CAD build for the part. Positions are in the model's coordinates, mm. A direction names the side the tool comes from. Coordinates: 2 decimals unless noted, no trailing zeros. Order: outer loops, then holes, each group sorted by start corner. A loop starts at its lowest first (then second) coordinate and runs counter-clockwise, first axis right, second up. Notation, with made-up numbers: (34, 0.5) - (88, 0.5) arc R8 cw to (88, 4.5) - close; hole circle Ø4 at (-39.75, 22). An arc over 180 degrees is marked (long way). Return JSON: item names as keys, results as strings.
from build123d import *

# Parameters (mm, degrees)
F0_W     = 30
F0_H     = 50
F1_DEPTH = 5
F2_W     = 23.511692
F2_H     = 14.549925
F2_R     = 5
F3_DEPTH = 3


with BuildPart() as f1:
    # F0 (on Front) → F1 (new body)
    with BuildSketch(Plane.XZ):
        Rectangle(F0_W, F0_H)
    extrude(amount=F1_DEPTH)

    # F2 (on face) → F3 (join)
    with BuildSketch(Plane.XZ.offset(5)):
        with Locations((0, 14.21516)):
            Rectangle(F2_W, F2_H)
        with Locations((-7.789027, -2.200567)):
            Circle(F2_R)
        with Locations((7.896153, -2.200567)):
            Circle(F2_R)
        with Locations((-7.789027, -14.839294)):
            Circle(F2_R)
        with Locations((7.896153, -14.839294)):
            Circle(F2_R)
    extrude(amount=F3_DEPTH)


solid = f1.part
Item 1: Wall check: L1, parallel to Z at x = 4, y = -5.75; L2, parallel to Z at x = 7.5, y = -6.5; L3, parallel to X at y = -7.25, z = 12. Give the ranges that are in metal, low to high. Write a range as [from, to].
Findings below:
{"L1": "z = [-17.97, -11.71], [-5.33, 0.93], [6.94, 21.49]", "L2": "z = [-19.82, -9.86], [-7.18, 2.78], [6.94, 21.49]", "L3": "x = [-11.76, 11.76]"}
Item 2: Which spindle directions (+Z, -Z, +X, -X, +Y, -Y) get a long thin tool onto all of the face, cutting with end or side? Do faces 1 (the flat face through (0, -6, 6.94)), 2 (the flat face through (11.756, -6, 14)), 3 (the flat face through (0, -6, 21.49)), 4 (the cylindrical face through (-12.784, -6.479, -1.981)). Say none if no direction does.
Findings below:
{"face 1": "+X, -X, -Y", "face 2": "+Z, +X, -Y", "face 3": "+Z, +X, -X, -Y", "face 4": "-Y"}
Item 3: Drop flat-ended pins along their axis: P1, Ø8, axis at x = 5, z = 6.5, coming from the -Y side; P2, Ø2.5, axis at y = -7, z = 16, coming from the +X side; P3, Ø1.5, axis at x = -3, y = -7, coming from the +Z side; P4, Ø1, axis at x = -0.5, z = -19.5, coming from the -Y side. Give the stop position or say it passes through.
Findings below:
{"P1": "stops at y = -8", "P2": "stops at x = 11.76", "P3": "stops at z = 21.49", "P4": "stops at y = -5"}
Item 4: Mould opens along X. For faces 5 (the flat face through (-8, -8, -15)), 6 (the cylindrical face through (-12.784, -6.479, -14.619)), 7 (the flat face through (-11.756, -6, 14)) say: released by +X, released by -X, zero draft, split by the parting line, or undercut.
Findings below:
{"face 5": "zero draft", "face 6": "undercut", "face 7": "released by -X"}
Item 5: Band-saw the part on C-C, the plane y = -6.75. List the corners of the cut face in (x, z), then the cut area to 3 significant figures.
Findings below:
{"outline": "circle Ø10 at (-7.79, -14.84); circle Ø10 at (-7.79, -2.2); (-11.76, 6.94) - (11.76, 6.94) - (11.76, 21.49) - (-11.76, 21.49) - close; circle Ø10 at (7.9, -14.84); circle Ø10 at (7.9, -2.2)", "area": "656 mm²"}
Item 6: Band-saw the part on B-B, the plane x = 8. List the corners of the cut face in (y, z), then the cut area to 3 significant figures.
Findings below:
{"outline": "(-8, -19.84) - (-5, -19.84) - (-5, -25) - (0, -25) - (0, 25) - (-5, 25) - (-5, 21.49) - (-8, 21.49) - (-8, 6.94) - (-5, 6.94) - (-5, 2.8) - (-8, 2.8) - (-8, -7.2) - (-5, -7.2) - (-5, -9.84) - (-8, -9.84) - close", "area": "354 mm²"}
Item 7: Band-saw the part on A-A, the plane z = 19.5. List the corners of the cut face in (x, y).
Findings below:
{"outline": "(-15, -5) - (-11.76, -5) - (-11.76, -8) - (11.76, -8) - (11.76, -5) - (15, -5) - (15, 0) - (-15, 0) - close"}
Item 8: Band-saw the part on D-D, the plane x = 5. List the corners of the cut face in (y, z), then the cut area to 3 significant figures.
Findings below:
{"outline": "(-8, -18.92) - (-5, -18.92) - (-5, -25) - (0, -25) - (0, 25) - (-5, 25) - (-5, 21.49) - (-8, 21.49) - (-8, 6.94) - (-5, 6.94) - (-5, 1.88) - (-8, 1.88) - (-8, -6.28) - (-5, -6.28) - (-5, -10.76) - (-8, -10.76) - close", "area": "343 mm²"}
